The listing builds one solid part. Answer for the finished solid, in the listing's coordinates (mm). A direction names the side the tool comes from. Give positions to 0.01 mm unless a question says otherwise; leave off trailing zeros. Write each loop counter-clockwise with the first axis right and the second up, starting at its lowest first coordinate (ties: lowest second). Pieces come first, ordered by that corner, then holes. Notation, with made-up numbers: (59.25, 75.25) - (102.25, 75.25) arc R34 cw to (102.25, 109.25) - close; hole circle Ø6 at (29, 50). An arc over 180 degrees is marked (long way). Return JSON: item names as keys, results as strings.
from build123d import *

# Parameters (mm, degrees)
PAD_DEPTH       = 80
POCKET_DEPTH    = 78
POCKET001_DEPTH = 408.7079232475
POCKET002_DEPTH = 408.4326470939
SKETCH004_W     = 93.184578
SKETCH004_H     = 155.633668
SKETCH004_W_2   = 509.235046
SKETCH004_H_2   = 157.082754
POCKET003_DEPTH = 80.001
POCKET004_DEPTH = 12.001
SKETCH006_W     = 8
SKETCH006_H     = 8
POCKET005_DEPTH = 10
SKETCH007_W     = 8
SKETCH007_H     = 8
POCKET006_DEPTH = 10
SKETCH008_R     = 1.55
POCKET007_DEPTH = 12.001
FILLET_R        = 2
FILLET001_R     = 2
FILLET002_R     = 2


with BuildPart() as part:
    # Sketch → Pad (new body)
    with BuildSketch(Plane.XY):
        Polygon((450, 0), (450, 90), (356, 87.18), (355.64, 99.18), (343.64, 98.82), (344, 86.82), (6, 76.68), (5.64, 88.6800000001), (-6.36, 88.3200000001), (-6, 76.32), (-50, 75), (-50, 0), align=None)
    extrude(amount=PAD_DEPTH)

    # Sketch001 (on Face14 of Pad) → Pocket (cut)
    with BuildSketch(Plane.XY.offset(80)):
        Polygon((-50, 15), (-50, 74), (450, 74), (450, 0), (356, 2.82), (356.3, 12.82), (344.3, 13.18), (344, 3.18), (6, 13.32), (6.3, 23.32), (-5.7, 23.68), (-6, 13.68), align=None)
    extrude(amount=-POCKET_DEPTH, mode=Mode.SUBTRACT)

    # Sketch002 (on Face26 of Pocket) → Pocket001 (cut, through all)
    with BuildSketch(Plane(origin=(355.5953641722, -10.6678609252, 0), x_dir=(0.0299865091, 0.9995503035, 0), z_dir=(0.9995503035, -0.0299865091, 0))):
        with BuildLine():
            ThreePointArc((23.4984280855, 56), (19.9988591841, 57.4495689014), (21.4484280855, 53.95))
            ThreePointArc((21.4484280855, 53.95), (17.8329435114, 41), (21.4484280855, 28.05))
            ThreePointArc((21.4484280855, 28.05), (19.9988591841, 24.5504310986), (23.4984280855, 26))
            Line((23.4984280855, 26), (23.4984280855, 56))
        make_face()
    extrude(amount=-POCKET001_DEPTH, mode=Mode.SUBTRACT)

    # Sketch003 (on Face14 of Pocket001) → Pocket002 (cut, through all)
    with BuildSketch(Plane(origin=(358.2929363573, 10.7487880907, 0), x_dir=(-0.0299865091, 0.9995503035, 0), z_dir=(0.9995503035, 0.0299865091, 0))):
        with BuildLine():
            ThreePointArc((88.470997005, 56), (84.9714281036, 57.4495689014), (86.420997005, 53.95))
            ThreePointArc((86.420997005, 53.95), (82.8055124309, 41), (86.420997005, 28.05))
            ThreePointArc((86.420997005, 28.05), (84.9714281036, 24.5504310986), (88.470997005, 26))
            Line((88.470997005, 26), (88.470997005, 56))
        make_face()
    extrude(amount=-POCKET002_DEPTH, mode=Mode.SUBTRACT)

    # Sketch004 (on Face7 of Pocket002) → Pocket003 (cut, through all)
    with BuildSketch(Plane.XY.offset(80)):
        with Locations((-52.592289, 54.389678)):
            Rectangle(SKETCH004_W, SKETCH004_H)
        with Locations((260.617523, 52.795659)):
            Rectangle(SKETCH004_W_2, SKETCH004_H_2)
    extrude(amount=-POCKET003_DEPTH, mode=Mode.SUBTRACT)

    # Sketch005 (on Face3 of Pocket003) → Pocket004 (cut, through all)
    with BuildSketch(Plane(origin=(-6, 0, 0), x_dir=(0, -1, 0), z_dir=(-1, 0, 0))):
        Polygon((12.873752, 2), (-23.68, 2), (-23.68, 84.957535), (-97.468468, 84.957535), (-97.468468, -3.470766), (12.873752, -3.470766), align=None)
    extrude(amount=-POCKET004_DEPTH, mode=Mode.SUBTRACT)

    # Sketch006 (on Face4 of Pocket004) → Pocket005 (cut)
    with BuildSketch(Plane.XY.offset(80)):
        with Locations((0, 14)):
            Rectangle(SKETCH006_W, SKETCH006_H)
    extrude(amount=-POCKET005_DEPTH, mode=Mode.SUBTRACT)

    # Sketch007 (on Face2 of Pocket005) → Pocket006 (cut)
    with BuildSketch(Plane(origin=(0, 0, 2), x_dir=(1, 0, 0), z_dir=(0, 0, -1))):
        with Locations((0, -14)):
            Rectangle(SKETCH007_W, SKETCH007_H)
    extrude(amount=-POCKET006_DEPTH, mode=Mode.SUBTRACT)

    # Sketch008 (on Face1 of Pocket006) → Pocket007 (cut, through all)
    with BuildSketch(Plane(origin=(-6, 0, 0), x_dir=(0, -1, 0), z_dir=(-1, 0, 0))):
        with Locations((-14, 8)):
            Circle(SKETCH008_R)
        with Locations((-14, 74)):
            Circle(SKETCH008_R)
        Polygon((-8, 22), (-8, 60), (0, 70), (0, 12), align=None)
    extrude(amount=-POCKET007_DEPTH, mode=Mode.SUBTRACT)

    # Fillet
    fillet_edges = [part.edges().sort_by_distance(p)[0] for p in [
        (-6, 8, 41),
    ]]
    fillet(fillet_edges, radius=FILLET_R)

    # Fillet001
    fillet001_edges = [part.edges().sort_by_distance(p)[0] for p in [
        (-6, 4, 65),
    ]]
    fillet(fillet001_edges, radius=FILLET001_R)

    # Fillet002
    fillet002_edges = [part.edges().sort_by_distance(p)[0] for p in [
        (-6, 4, 17),
    ]]
    fillet(fillet002_edges, radius=FILLET002_R)


solid = part.part
Item 1: Flat-ended cylindrical pins translate along their axes: P1, Ø2.5, axis at x = -2, z = 77, coming from the +Y side; P2, Ø4, axis at x = 1, z = 7.5, coming from the +Y side; P3, Ø8, axis at y = 5, z = 48, coming from the -X side. Find the tip coordinate at first contact, or state that the pin passes through.
Answer below:
{"P1": "stops at y = 23.61", "P2": "stops at y = 23.54", "P3": "stops at x = -5.73"}
Item 2: Consider L1, parallel to Z at x = 5.6, y = 14; L2, parallel to Z at x = 0.5, y = 20.5; L3, parallel to X at y = 12.5, z = 75. Determine where each line is inside the solid, lowest interval first.
Answer below:
{"L1": "z = 2 to 6.45, 9.55 to 72.45, 75.55 to 80", "L2": "z = 2 to 24.18, 27.82 to 29.75, 52.25 to 54.18, 57.82 to 80", "L3": "x = -6 to -4, 4 to 6"}
Item 3: For faces 1 (the face through (-5.4, 3.81, 15.85)), 2 (the face through (1, 4, 65)), 3 (the face through (-4, 14, 6)), 4 (the face through (4, 14, 76)), determine the directions among +Z, -Z, +X, -X, +Y, -Y from which every point of the face is accessible in a straight line to the end or side of a thin tool.
Answer below:
{"face 1": "-X, -Y", "face 2": "+X, -X, -Y", "face 3": "-Z", "face 4": "+Z"}
Item 4: A cutting plane is placed at A-A on z = 74. Determine the outline of the cut face in (x, y), then the cut area to 3 significant figures.
Answer below:
{"outline": "(-6, 0) - (6, 0) - (6, 12.45) - (4, 12.45) - (4, 10) - (-4, 10) - (-4, 12.45) - (-6, 12.45) - close; (-5.94, 15.55) - (-4, 15.55) - (-4, 18) - (4, 18) - (4, 15.55) - (6, 15.55) - (6, 23.33) - (-5.7, 23.68) - close", "area": "204 mm²"}
Item 5: The mould has two halves that part along Z. Classify faces 5 (the face through (-6, 11, 42)), 6 (the face through (0, 14, 12)), 7 (the face through (4.986, 14.202, 75.537)): +Z half, -Z half, draft (parallel to the pull), parting line (faces both ways), or undercut.
Answer below:
{"face 5": "draft", "face 6": "-Z half", "face 7": "undercut"}
Item 6: A cutting plane is placed at B-B on y = 11.5. Determine the outline of the cut face in (x, z).
Answer below:
{"outline": "(-6, 2) - (-4, 2) - (-4, 12) - (4, 12) - (4, 2) - (6, 2) - (6, 80) - (4, 80) - (4, 70) - (-4, 70) - (-4, 80) - (-6, 80) - close"}
Item 7: A cutting plane is placed at C-C on z = 40.5. Determine the outline of the cut face in (x, y), then the cut area to 3 significant figures.
Answer below:
{"outline": "(-6, 10) arc R2 ccw to (-4, 8) - (6, 8) - (6, 17.67) - (-5.87, 18.02) - (-6, 13.68) - close", "area": "117 mm²"}
